Build history of the part. All positions in model axes, mm. Face numbers are marked on the shaded views. Give positions to 0.01 mm unless a question says otherwise; leave off trailing zeros. Loops run counter-clockwise (first coordinate to the right, second up) from the corner with the lowest first, then second, coordinate; pieces in that order, holes last. Notation, with made-up numbers: (-1.5, 75.5) -> (9.5, 75.5) arc R21 cw to (9.5, 98.5) -> close; hole circle Ø10 at (70.25, 47.5). An arc over 180 degrees is marked (long way). Answer as a JSON object with one key per item and string values. Group by question number.
Q1. Band-saw the part on C-C, the plane x = 20. Write the cut outline in (y, z).
Q2. Drop flat-ended pins along their axis: pin 1 (10 mm diameter, centred on x = 15, z = 15.5, fed in from -Y); pin 2 (1 mm diameter, centred on y = 3.5, z = 15.5, fed in from +X); pin 3 (1 mm diameter, centred on y = 16.5, z = 16.5, fed in from +X); pin 4 (8 mm diameter, centred on x = 19.5, y = 16.5, fed in from -Z). Give the stop position or say it passes through.
Q3. Wall check: probe 1 along Y at (x, z) = (0, 34.05); probe 2 along Y at (x, z) = (0, 1.3); probe 3 along X at (y, z) = (0.5, 10.5). Give the ranges that are in metal, low to high. Write a range as from..to.
Q4. Band-saw the part on D-D, the plane z = 9. Write the cut outline in (x, y).
Q5. Band-saw the part on A-A, the plane y = 0. Write the cut outline in (x, z), plus the area to 3 significant figures.
Q6. Two-plate mould, pull along X, no slides. Class the marked faces 1, 2, 3 and 4: pulls with the +X half, pulls with the -X half, needs draft (parallel to the pull), parting line crosses it, or undercut.
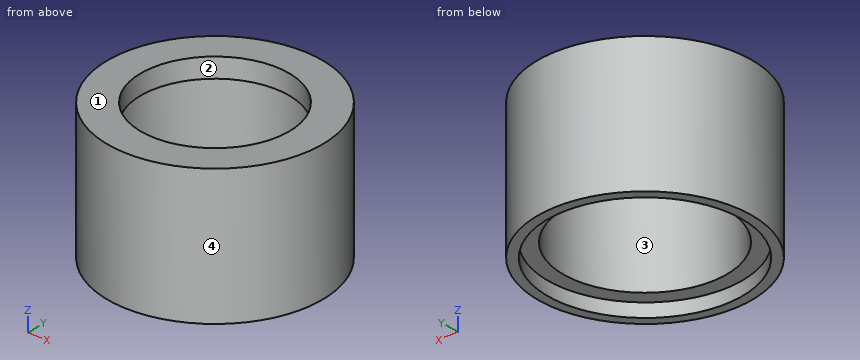
from build123d import *

# Parameters (mm, degrees)
SKETCH_1_R          = 27.5
EXTRUDE_1_DEPTH     = 3
SKETCH_2_R          = 27.5
EXTRUDE_2_DEPTH     = 32
SKETCH_3_R          = 21
CUT_EXTRUDE_1_DEPTH = 30
SKETCH_4_R          = 19
CUT_EXTRUDE_2_DEPTH = 30
SKETCH_5_R          = 25
CUT_EXTRUDE_3_DEPTH = 3.5


with BuildPart() as part:
    # 草图1 → 拉伸1 (new body)
    with BuildSketch(Plane.XY):
        Circle(SKETCH_1_R)
    extrude(amount=EXTRUDE_1_DEPTH)

    # 草图2 → 拉伸2 (add)
    with BuildSketch(Plane.XY.offset(3)):
        Circle(SKETCH_2_R)
    extrude(amount=EXTRUDE_2_DEPTH)

    # 草图3 → 切除-拉伸1 (cut)
    with BuildSketch(Plane(origin=(0, 0, 0), x_dir=(-1, 0, 0), z_dir=(0, 0, -1))):
        Circle(SKETCH_3_R)
    extrude(amount=-CUT_EXTRUDE_1_DEPTH, mode=Mode.SUBTRACT)

    # 草图4 → 切除-拉伸2 (cut)
    with BuildSketch(Plane(origin=(0, 0, 30), x_dir=(-1, 0, 0), z_dir=(0, 0, -1))):
        Circle(SKETCH_4_R)
    extrude(amount=-CUT_EXTRUDE_2_DEPTH, mode=Mode.SUBTRACT)

    # 草图5 → 切除-拉伸3 (cut)
    with BuildSketch(Plane(origin=(0, 0, 0), x_dir=(-1, 0, 0), z_dir=(0, 0, -1))):
        Circle(SKETCH_5_R)
    extrude(amount=-CUT_EXTRUDE_3_DEPTH, mode=Mode.SUBTRACT)


solid = part.part
Worked answers:
{
 "1": {"outline": "(-18.87, 0) -> (-15, 0) -> (-15, 3.5) -> (-6.4, 3.5) -> (-6.4, 30) -> (6.4, 30) -> (6.4, 3.5) -> (15, 3.5) -> (15, 0) -> (18.87, 0) -> (18.87, 35) -> (-18.87, 35) -> close"},
 "2": {"pin 1": "y = -25.62", "pin 2": "x = 27.34", "pin 3": "x = 22.37", "pin 4": "z = 0"},
 "3": {"probe 1": "-27.5..-19, 19..27.5", "probe 2": "-27.5..-25, 25..27.5", "probe 3": "-27.5..-20.99, 20.99..27.5"},
 "4": {"outline": "circle Ø55 at (0, 0); hole circle Ø42 at (0, 0)"},
 "5": {"outline": "(-27.5, 0) -> (-25, 0) -> (-25, 3.5) -> (-21, 3.5) -> (-21, 30) -> (-19, 30) -> (-19, 35) -> (-27.5, 35) -> close; (19, 30) -> (21, 30) -> (21, 3.5) -> (25, 3.5) -> (25, 0) -> (27.5, 0) -> (27.5, 35) -> (19, 35) -> close", "area": "447 mm2"},
 "6": {"face 1": "needs draft", "face 2": "undercut", "face 3": "undercut", "face 4": "parting line crosses it"}
}
